Work out the finished part from the listing and answer in its coordinate system (mm). A direction names the side the tool comes from. Coordinates: 2 decimals unless noted, no trailing zeros. Order: outer loops, then holes, each group sorted by start corner. A loop starts at its lowest first (then second) coordinate and runs counter-clockwise, first axis right, second up.
1. The part is cut by section C-C, the plane x = 0. Give the vertices of the cut face in (y, z).
2. A tool of negligible diameter and unlimited length cuts with its end or side. For faces 1 (the cylindrical face through (14.22, 16.41, 2.46)), 2 (the flat face through (-18, 2.4, 4)), from which of +Z, -Z, +X, -X, +Y, -Y can it reach the whole face along a straight path? Write none if from no direction.
3. Determine the mould class of faces 3 (the flat face through (0, 14, 5)), 4 (the cylindrical face through (23.556, -9.767, 2.465)), 5 (the flat face through (18, 0, 2.5)) for opening direction Y: +Y half, -Y half, draft (parallel to the pull), parting line (faces both ways), or undercut.
4. The part is cut by section B-B, the plane z = 3.8. Give the vertices of the cut face in (x, y) (3 decimals), then the cut area to 3 significant figures.
5. Flat-ended cylindrical pins translate along their axes: pin 1 Ø2 at (x, z) = (-4, 1) entering from +Y; pin 2 Ø3 at (x, z) = (18.5, 3.5) entering from -Y; pin 3 Ø3.5 at (x, y) = (14.475, -14.475) entering from -Z; pin 4 Ø2.5 at (x, y) = (-18, -1) entering from +Z. Find the tip coordinate at first contact, or state that the pin passes through.
6. The part is cut by section D-D, the plane x = 14.5. Give the vertices of the cut face in (y, z).
7. The part is cut by section A-A, the plane y = 0. Give the vertices of the cut face in (x, z).
8. Find the intervals of material crossed by probe 1 along Y at (x, z) = (0, 1.4); probe 2 along Y at (x, z) = (-16.5, 4.3); probe 3 along Y at (x, z) = (-19.5, 1.45), in increasing order.
```python
from build123d import *

# Parameters (mm, degrees)
F0_R     = 25.5
F0_R_2   = 1.95
F0_R_3   = 10.71
F1_DEPTH = 5
F3_DEPTH = 2.5


with BuildPart() as f1:
    # F0 (on Top) → F1 (new body)
    with BuildSketch(Plane.XY):
        Circle(F0_R)
        with Locations((-14.475, -14.475)):
            Circle(F0_R_2, mode=Mode.SUBTRACT)
        with Locations((14.475, -14.475)):
            Circle(F0_R_2, mode=Mode.SUBTRACT)
        with Locations((-14.475, 14.475)):
            Circle(F0_R_2, mode=Mode.SUBTRACT)
        Circle(F0_R_3, mode=Mode.SUBTRACT)
        with Locations((14.475, 14.475)):
            Circle(F0_R_2, mode=Mode.SUBTRACT)
    extrude(amount=F1_DEPTH)

    # F2 (on face) → F3 (cut)
    with BuildSketch(Plane.XY.offset(5)):
        with BuildLine():
            Line((-10.4376290411, 2.4), (-25.3868075976, 2.4))
            ThreePointArc((-25.3868075976, 2.4), (-25.4716861803, 1.2013338961), (-25.5, 0))
            ThreePointArc((-25.5, 0), (-25.4716861803, -1.2013338961), (-25.3868075976, -2.4))
            Line((-25.3868075976, -2.4), (-10.4376290411, -2.4))
            ThreePointArc((-10.4376290411, -2.4), (-10.71, 0), (-10.4376290411, 2.4))
        make_face()
        with BuildLine():
            ThreePointArc((25.5, 0), (25.4716861803, 1.2013338961), (25.3868075976, 2.4))
            Line((25.3868075976, 2.4), (10.4376290411, 2.4))
            ThreePointArc((10.4376290411, 2.4), (10.6416894108, 1.2077029787), (10.71, 0))
            ThreePointArc((10.71, 0), (10.6416894108, -1.2077029787), (10.4376290411, -2.4))
            Line((10.4376290411, -2.4), (25.3868075976, -2.4))
            ThreePointArc((25.3868075976, -2.4), (25.4716861803, -1.2013338961), (25.5, 0))
        make_face()
    extrude(amount=-F3_DEPTH, mode=Mode.SUBTRACT)


solid = f1.part
```
Geometry says:
1. outline: (-25.5, 0) - (-10.71, 0) - (-10.71, 5) - (-25.5, 5) - close; (10.71, 0) - (25.5, 0) - (25.5, 5) - (10.71, 5) - close
2. face 1: +Z, -Z
2. face 2: +Z, +X, -X
3. face 3: draft
3. face 4: parting line
3. face 5: undercut
4. outline: (-25.387, -2.4) arc R25.5 ccw to (25.387, -2.4) - (10.438, -2.4) arc R10.71 cw to (-10.438, -2.4) - close; (-25.387, 2.4) - (-10.438, 2.4) arc R10.71 cw to (10.438, 2.4) - (25.387, 2.4) arc R25.5 ccw to start; hole circle Ø3.9 at (-14.475, -14.475); hole circle Ø3.9 at (-14.475, 14.475); hole circle Ø3.9 at (14.475, -14.475); hole circle Ø3.9 at (14.475, 14.475)
4. area: 1,490 mm2
5. pin 1: stops at y = 25.32
5. pin 2: stops at y = -19.01
5. pin 3: passes through
5. pin 4: stops at z = 2.5
6. outline: (-20.98, 0) - (-16.42, 0) - (-16.42, 5) - (-20.98, 5) - close; (-12.53, 0) - (12.53, 0) - (12.53, 5) - (2.4, 5) - (2.4, 2.5) - (-2.4, 2.5) - (-2.4, 5) - (-12.53, 5) - close; (16.42, 0) - (20.98, 0) - (20.98, 5) - (16.42, 5) - close
7. outline: (-25.5, 0) - (-10.71, 0) - (-10.71, 2.5) - (-25.5, 2.5) - close; (10.71, 0) - (25.5, 0) - (25.5, 2.5) - (10.71, 2.5) - close
8. probe 1: y = -25.5 to -10.71, 10.71 to 25.5
8. probe 2: y = -19.44 to -2.4, 2.4 to 19.44
8. probe 3: y = -16.43 to 16.43
